Can you work these out from the model? Positions are in its coordinate system, mm. A direction names the side the tool comes from. Give positions to 0.01 mm unless a question says otherwise; leave off trailing zeros. Write each loop counter-clockwise with the first axis right and the second up, starting at its lowest first coordinate (ties: lowest second). Pieces come first, ordered by that corner, then holes. Notation, with made-up numbers: (61.25, 24) -> (79.25, 24) arc R27 cw to (79.25, 61) -> close; hole circle Ø9 at (3, 34.5). An arc over 180 degrees is marked (long way). One line per item, written item: value.
from build123d import *

# Parameters (mm, degrees)
SKETCH_1_R                 = 2.9
EXTRUDE_1_DEPTH            = 30
SKETCH_2_W                 = 27.5
SKETCH_2_H                 = 30
EXTRUDE_2_DEPTH            = 17
CUT_EXTRUDE_1_REACH        = 39.833
SKETCH_3_W                 = 27.5
SKETCH_3_H                 = 19.8
SKETCH_4_W                 = 27.5
SKETCH_4_H                 = 30
SKETCH_4_W_2               = 23
SKETCH_4_H_2               = 27.5
CUT_EXTRUDE_2_DEPTH        = 4.5
CHAMFER_1_SIZE             = 3
SKETCH_5_W                 = 20.5
SKETCH_5_H                 = 13
CUT_EXTRUDE_3_DEPTH        = 3
SKETCH_6_R                 = 7.5
SKETCH_6_R_2               = 2.9
EXTRUDE_3_DEPTH            = 2.2
CHAMFER_2_SIZE             = 2
CHAMFER_2_OF_MIRROR_1_SIZE = 2


with BuildPart() as part:
    # 草图1 → 凸台-拉伸1 (new body)
    with BuildSketch(Plane(origin=(0, 0, 0), x_dir=(1, 0, 0), z_dir=(0, 1, 0))):
        with BuildLine():
            Line((-0.305751289, 8.694625705), (9.8, 9.05))
            Line((9.8, 9.05), (9.8, -9.05))
            Line((9.8, -9.05), (-0.305751289, -8.694625705))
            ThreePointArc((-0.305751289, -8.694625705), (-8.7, 0), (-0.305751289, 8.694625705))
        make_face()
        with Locations(Location((0, 0, 0), (0, 0, 270))):
            Circle(SKETCH_1_R, mode=Mode.SUBTRACT)
    extrude(amount=EXTRUDE_1_DEPTH)

    # 草图2 → 凸台-拉伸2 (add)
    with BuildSketch(Plane(origin=(9.8, 0, 0), x_dir=(0, 0, -1), z_dir=(1, 0, 0))):
        with Locations((0, 15)):
            Rectangle(SKETCH_2_W, SKETCH_2_H)
    extrude(amount=EXTRUDE_2_DEPTH)

    # 草图3 → 切除-拉伸1 (cut, up to next)
    with BuildSketch(Plane.ZY.offset(-9.8), mode=Mode.PRIVATE) as cut_extrude_1_sk1:
        with Locations((0, 15)):
            Rectangle(SKETCH_3_W, SKETCH_3_H)
    cut_extrude_1_tool1 = extrude(cut_extrude_1_sk1.sketch, amount=CUT_EXTRUDE_1_REACH, mode=Mode.PRIVATE) & part.part
    add(cut_extrude_1_tool1.solids().sort_by_distance((9.8, 15, 0))[0], mode=Mode.SUBTRACT)

    # 草图4 → 切除-拉伸2 (cut)
    with BuildSketch(Plane(origin=(26.8, 0, 0), x_dir=(0, 0, -1), z_dir=(1, 0, 0))):
        with Locations((0, 15)):
            Rectangle(SKETCH_4_W, SKETCH_4_H)
        with Locations((0, 15)):
            Rectangle(SKETCH_4_W_2, SKETCH_4_H_2, mode=Mode.SUBTRACT)
    extrude(amount=-CUT_EXTRUDE_2_DEPTH, mode=Mode.SUBTRACT)

    # 倒角1
    chamfer_1_edges = [part.edges().sort_by_distance(p)[0] for p in [
        (26.8, 15, -11.5),
    ]]
    chamfer(chamfer_1_edges, length=CHAMFER_1_SIZE)

    # 草图5 → 切除-拉伸3 (cut)
    with BuildSketch(Plane(origin=(26.8, 0, 0), x_dir=(0, 0, -1), z_dir=(1, 0, 0))):
        with Locations((1.25, 15)):
            Rectangle(SKETCH_5_W, SKETCH_5_H)
    extrude(amount=-CUT_EXTRUDE_3_DEPTH, mode=Mode.SUBTRACT)

    # 草图6 → 凸台-拉伸3 (add)
    with BuildSketch(Plane(origin=(0, 30, 0), x_dir=(1, 0, 0), z_dir=(0, 1, 0))):
        with Locations(Location((0, 0, 0), (0, 0, 270))):
            Circle(SKETCH_6_R)
        with Locations(Location((0, 0, 0), (0, 0, 270))):
            Circle(SKETCH_6_R_2, mode=Mode.SUBTRACT)
    extrude_3 = extrude(amount=EXTRUDE_3_DEPTH)

    # 倒角2
    chamfer_2_edges = [part.edges().sort_by_distance(p)[0] for p in [
        (0, 32.2, -7.5),
    ]]
    chamfer(chamfer_2_edges, length=CHAMFER_2_SIZE)

    # 镜向1: 凸台-拉伸3 across plane
    add(extrude_3.mirror(Plane(origin=(0, 15, 0), x_dir=(0, 0, 1), z_dir=(0, -1, 0))))

    # 倒角2 of 镜向1
    chamfer_2_of_mirror_1_edges = [part.edges().sort_by_distance(p)[0] for p in [
        (0, -2.2, -7.5),
    ]]
    chamfer(chamfer_2_of_mirror_1_edges, length=CHAMFER_2_OF_MIRROR_1_SIZE)


solid = part.part
1) If we section it at A-A (y = 2.5): Write out the boundary of the cut face in (x, z).
Answer list:
outline: (-0.31, -8.69) -> (9.8, -9.05) -> (9.8, -13.75) -> (22.3, -13.75) -> (22.3, -11.5) -> (23.8, -11.5) -> (26.8, -8.5) -> (26.8, 11.5) -> (22.3, 11.5) -> (22.3, 13.75) -> (9.8, 13.75) -> (9.8, 9.05) -> (-0.31, 8.69) arc R8.7 ccw to start; hole circle Ø5.8 at (0, 0)
2) I need wall thicknesses on L1, parallel to Y at x = 8.5, z = -4; L2, parallel to Y at x = 24.5, z = -10; L3, parallel to Z at x = 0, y = 29. Which ranges of each line are inside material? Lowest first, please.
Answer list:
L1: y = 0 to 5.1, 24.9 to 30
L2: y = 1.25 to 8.5, 21.5 to 28.75
L3: z = -8.71 to -2.9, 2.9 to 8.71
3) If we section it at C-C (y = 6.5): Write out the boundary of the cut face in (x, z), and give its area (3 significant figures).
Answer list:
outline: (9.8, -13.75) -> (22.3, -13.75) -> (22.3, -11.5) -> (23.8, -11.5) -> (26.8, -8.5) -> (26.8, 11.5) -> (22.3, 11.5) -> (22.3, 13.75) -> (9.8, 13.75) -> close
area: 443 mm^2
4) For faces 4 (the face through (25, 8.5, -1)), 5 (the face through (16, 15, 13.75)), 6 (the face through (25.3, 4.8, -10)), 7 (the face through (3, 24.9, 2)), 8 (the face through (25, 28.75, 0)), which set-ups out of +Z, -Z, +X, -X, +Y, -Y let a thin tool reach every point of the face, with its end or its side?
Answer list:
face 4: -Z, +X
face 5: +Z, +X, -X, +Y, -Y
face 6: -Z, +X, +Y, -Y
face 7: +Z, -Z, -X
face 8: +Z, -Z, +X, +Y
5) If we section it at B-B (z = 10.5): Write out the boundary of the cut face in (x, y), and give its area (3 significant figures).
Answer list:
outline: (9.8, 0) -> (22.3, 0) -> (22.3, 1.25) -> (26.8, 1.25) -> (26.8, 28.75) -> (22.3, 28.75) -> (22.3, 30) -> (9.8, 30) -> close
area: 499 mm^2
6) We'd pull the mould along Z, two halves only. Please class faces 1 (the face through (3, 5.1, 2)), 2 (the face through (16, 15, -13.75)), 3 (the face through (0.1, 28.5, -2.9)): released by +Z, released by -Z, zero draft, split by the parting line, or undercut.
Answer list:
face 1: zero draft
face 2: released by -Z
face 3: undercut
7) Will these pins go through, and if not, where does the flat tip stop? pin 1 (3 mm diameter, centred on x = 1.5, y = 23.5, fed in from +Z); pin 2 (6.5 mm diameter, centred on x = 0, z = 0, fed in from +Y); pin 3 (5 mm diameter, centred on x = 15, z = -11, fed in from -Y); pin 4 (0.9 mm diameter, centred on x = 25, z = -2.5, fed in from +Y).
Answer list:
pin 1: stops at z = 8.78
pin 2: stops at y = 32.2
pin 3: stops at y = 0
pin 4: stops at y = 28.75
8) If we section it at D-D (x = 21.5): Write out the boundary of the cut face in (y, z), and give its area (3 significant figures).
Answer list:
outline: (0, -13.75) -> (30, -13.75) -> (30, 13.75) -> (0, 13.75) -> close
area: 825 mm^2
